Part model, mm, in its own coordinate system. Round coordinates to 2 decimals unless told otherwise and drop trailing zeros. Write each loop counter-clockwise with the first axis right and the second up, starting at its lowest first coordinate (ties: lowest second). Pieces come first, ordered by that corner, then holes. Notation, with made-up numbers: M -29,82 L -24,82 A32 ccw -24,113 Z; hole C 70.5,-16 d1. An arc over 180 degrees is marked long. Use a Markdown table: item, result. Add a question column.
1) Slice it at D-D on z = -50. Write the cut outline in (x, y), plus the area to 3 significant figures.
2) Drop flat-ended pins along their axis: P1, Ø4, axis at x = 563.5, y = 7.5, coming from the -Z side; P2, Ø3, axis at y = -49, z = 23.5, coming from the -X side; P3, Ø2, axis at x = 325, z = -2, coming from the +Y side. Give the stop position or say it passes through.
3) Slice it at C-C on z = 61.5. Write the cut outline in (x, y).
4) Two-plate mould, pull along X, no slides. Class faces 1 (the face through (-9, 0, 0)), 2 (the face through (-22.453, 4.986, 49.3)), 3 (the face through (245.951, 22.804, 2.994)), 4 (the face through (0, 0, -9)): released by +X, released by -X, zero draft, split by the parting line, or undercut.
5) Wall check: probe 1 along Y at (x, z) = (490.5, 1.5); probe 2 along Z at (x, y) = (153.5, -0.5); probe 3 along X at (y, z) = (5, 31). Give the ranges that are in metal, low to high.
6) Slice it at A-A on y = 0. Write the cut outline in (x, z), plus the area to 3 significant figures.
7) Slice it at B-B on x = 382. Write the cut outline in (y, z).
```python
from build123d import *

# Parameters (mm, degrees)
SKETCH1_R       = 23
LENGTH_DEPTH    = 565
SKETCH2_R       = 23
HIP_JOINT_DEPTH = 100


with BuildPart() as part:
    # Sketch1 → Length (new body)
    with BuildSketch(Plane(origin=(0, 0, 0), x_dir=(0, 0, -1), z_dir=(1, 0, 0))):
        Circle(SKETCH1_R)
    extrude(amount=LENGTH_DEPTH)

    # Sketch2 → Hip joint (add)
    with BuildSketch(Plane.XY):
        with Locations(Location((0, 0, 0), (0, 0, 270))):
            Circle(SKETCH2_R)
    extrude(amount=HIP_JOINT_DEPTH)

    # Sketch10 → Revolve23 (revolve)
    with BuildSketch(Plane.XY):
        with BuildLine():
            Line((495, 0), (635, 0))
            ThreePointArc((635, 0), (565, -70), (495, 0))
        make_face()
    revolve(axis=Axis((565, 0, 0), (-1, 0, 0)))


solid = part.part
```
Entries:
| question | item | result |
|---|---|---|
| 1 | outline | C 565,0 d97.98 |
| 1 | area | 7,540 mm^2 |
| 2 | P1 | stops at z = -69.77 |
| 2 | P2 | stops at x = 519.09 |
| 2 | P3 | stops at y = 22.98 |
| 3 | outline | C 0,0 d46; C 565,0 d66.87 |
| 4 | face 1 | zero draft |
| 4 | face 2 | undercut |
| 4 | face 3 | undercut |
| 4 | face 4 | released by -X |
| 5 | probe 1 | y = -22.95 to 22.95 |
| 5 | probe 2 | z = -22.99 to 22.99 |
| 5 | probe 3 | x = -22.45 to 22.45, 502.44 to 627.56 |
| 6 | outline | M -23,0 L 0,0 L 0,-23 L 498.89,-23 A70 ccw long 498.89,23 L 23,23 L 23,100 L -23,100 Z |
| 6 | area | 42,300 mm^2 |
| 7 | outline | C 0,0 d46 |
